```python
from build123d import *

# Parameters (mm, degrees)
EXTRUDE_1_DEPTH       = 30
SKETCH_2_R            = 15
CUT_EXTRUDE_2_DEPTH   = 45.532745299
EXTRUDE_3_DEPTH       = 45
CUT_EXTRUDE_START     = 70
SKETCH_3_W            = 44.656689001
SKETCH_3_H            = 20
CUT_EXTRUDE_1_DEPTH   = 130
SKETCH_7_R            = 3.999999997
CUT_EXTRUDE_2_2_DEPTH = 81.051544881
FILLET_1_R            = 5
CHAMFER_5_SIZE        = 2
CHAMFER_6_SIZE        = 10


with BuildPart() as part:
    # Эскиз1 → Вытянуть1 (new body)
    with BuildSketch(Plane(origin=(0, 0, 0), x_dir=(1, 0, 0), z_dir=(0, 1, 0))):
        Polygon((-24.019063342, 22.5), (10.980936658, 22.5), (19.22346273, 15), (19.22346273, -15), (10.980936658, -22.5), (-24.019063342, -22.5), align=None)
    extrude(amount=EXTRUDE_1_DEPTH)

    # Эскиз2 → Cut-Extrude 2 (cut, through all)
    with BuildSketch(Plane(origin=(0, 30, 0), x_dir=(1, 0, 0), z_dir=(0, 1, 0))):
        with Locations(Location((0, 0, 0), (0, 0, 270))):
            Circle(SKETCH_2_R)
    extrude(amount=-CUT_EXTRUDE_2_DEPTH, mode=Mode.SUBTRACT)

    # Эскиз6 → Вытянуть3 (add)
    with BuildSketch(Plane(origin=(0, 0, -22.5), x_dir=(-1, 0, 0), z_dir=(0, 0, -1))):
        Polygon((24.019063342, -19.927530698), (24.019063342, 30), (59.019063342, 6.012561534), (59.019063342, -19.927530698), align=None)
    extrude(amount=-EXTRUDE_3_DEPTH)

    # Эскиз3 → Вырез-Вытянуть1 (cut)
    with BuildSketch(Plane(origin=(0, 30, 0), x_dir=(1, 0, 0), z_dir=(0, 1, 0)).offset(CUT_EXTRUDE_START)):
        with Locations((-43.210774099, 0)):
            Rectangle(SKETCH_3_W, SKETCH_3_H)
    extrude(amount=-CUT_EXTRUDE_1_DEPTH, mode=Mode.SUBTRACT)

    # Эскиз7 → Cut-Extrude 2 2 (cut, through all)
    with BuildSketch(Plane(origin=(0, 0, -22.5), x_dir=(-1, 0, 0), z_dir=(0, 0, -1))):
        with Locations((41.170494395, -12.547441244)):
            Circle(SKETCH_7_R)
    extrude(amount=-CUT_EXTRUDE_2_2_DEPTH, mode=Mode.SUBTRACT)

    # Скругление1
    fillet_1_edges = [part.edges().sort_by_distance(p)[0] for p in [
        (-24.019063342, 0, -16.25),
    ]]
    fillet(fillet_1_edges, radius=FILLET_1_R)

    # Фаска5
    chamfer_5_edges = [part.edges().sort_by_distance(p)[0] for p in [
        (-59.019063342, -19.927530698, 16.25),
        (-59.019063342, -19.927530698, -16.25),
    ]]
    chamfer(chamfer_5_edges, length=CHAMFER_5_SIZE)

    # Фаска6
    chamfer_6_edges = [part.edges().sort_by_distance(p)[0] for p in [
        (-24.019063342, -19.927530698, 16.25),
        (-24.019063342, -19.927530698, -16.25),
    ]]
    chamfer(chamfer_6_edges, length=CHAMFER_6_SIZE)


solid = part.part
```
For this review, take the finished solid that the model builds, in its own axes (mm). A direction names the side the tool comes from. Coordinates: 2 decimals unless noted, no trailing zeros. Loops run counter-clockwise (first coordinate to the right, second up) from the corner with the lowest first, then second, coordinate; pieces in that order, holes last. Notation, with made-up numbers: (32, 67) -> (62, 67) arc R12 ccw to (62, 79) -> close; hole circle Ø3 at (76, 54). An arc over 180 degrees is marked (long way). Return JSON: item names as keys, results as strings. Group by question number.
(1) Consider section A-A, the plane z = 11. Give the boundary of the cut face in (x, y).
(2) Consider section B-B, the plane x = 0. Give the boundary of the cut face in (y, z), plus the area to 3 significant figures.
(3) Consider section D-D, the plane z = 0. Give the boundary of the cut face in (x, y).
(4) For pin 1 Ø2.5 at (y, z) = (-7, 18) entering from +X; pin 2 Ø1 at (y, z) = (11.5, -7.5) entering from -X; pin 3 Ø7 at (x, y) = (-41.17, -12.55) entering from +Z, all flat-tipped, find the tip position at first contact; note any pin that passes through.
(5) To check wall thickness, follow L1, parallel to X at y = 8.5, z = 0; L2, parallel to Z at x = -25, y = 3; L3, parallel to Y at x = -8, z = 13. State the ranges of each line that lie inside material, in increasing order.
(6) Tool access review of faces 5 (the flat face through (-20.882, 15, 0)), 6 (the flat face through (19.223, 15, 0)), 7 (the flat face through (0.4, 0, -15.3)): name each direction out of +Z, -Z, +X, -X, +Y, -Y from which nothing blocks a thin tool from reaching the whole face with its end or side.
(7) Consider section C-C, the plane y = -6.5. Give the boundary of the cut face in (x, z).
(8) Mouldability with a two-part tool opening along Y and no side actions: class faces 1 (the cylindrical face through (-37.174, -12.372, -16.337)), 2 (the cylindrical face through (-20.366, -0.185, -0.315)), 3 (the flat face through (-40, 0, 10)), 4 (the cylindrical face through (-37.174, -12.372, 16.163)) as pulls with the +Y half, pulls with the -Y half, needs draft (parallel to the pull), parting line crosses it, or undercut.
Results below:
{
 "1": {"outline": "(-59.02, -17.93) -> (-57.02, -19.93) -> (-34.02, -19.93) -> (-24.02, -9.93) -> (-24.02, -5) arc R5 cw to (-19.02, 0) -> (-10.2, 0) -> (-10.2, 30) -> (-24.02, 30) -> (-59.02, 6.01) -> close; (10.2, 0) -> (19.22, 0) -> (19.22, 30) -> (10.2, 30) -> close; hole circle Ø8 at (-41.17, -12.55)"},
 "2": {"outline": "(0, -22.5) -> (30, -22.5) -> (30, -15) -> (0, -15) -> close; (0, 15) -> (30, 15) -> (30, 22.5) -> (0, 22.5) -> close", "area": "450 mm2"},
 "3": {"outline": "(-20.88, -0.36) arc R5 cw to (-19.02, 0) -> (-15, 0) -> (-15, 30) -> (-20.88, 30) -> close; (15, 0) -> (19.22, 0) -> (19.22, 30) -> (15, 30) -> close"},
 "4": {"pin 1": "stops at x = -24.02", "pin 2": "stops at x = -20.88", "pin 3": "passes through"},
 "5": {"L1": "x = -20.88 to -15, 15 to 19.22", "L2": "z = -22.5 to -10, 10 to 22.5", "L3": "y = 0 to 30"},
 "6": {"face 5": "-X, +Y, -Y", "face 6": "+Z, -Z, +X, +Y, -Y", "face 7": "+Z, -Z, +X, -Y"},
 "7": {"outline": "(-59.02, -22.5) -> (-24.02, -22.5) -> (-24.02, -10) -> (-59.02, -10) -> close; (-59.02, 10) -> (-24.02, 10) -> (-24.02, 22.5) -> (-59.02, 22.5) -> close"},
 "8": {"face 1": "undercut", "face 2": "pulls with the -Y half", "face 3": "needs draft", "face 4": "undercut"}
}
